```python
from build123d import *

# Parameters (mm, degrees)
SKETCH1_R           = 8.25
BOSS_EXTRUDE1_DEPTH = 85
SKETCH2_OUTSIDE_W   = 36.128
SKETCH2_OUTSIDE_H   = 36.128
SKETCH2_OUTSIDE_R   = 2
CUT_EXTRUDE1_DEPTH  = 12
SKETCH3_R           = 4.75
SKETCH3_R_2         = 4.25
BOSS_EXTRUDE2_DEPTH = 10
CHAMFER1_SIZE       = 1
CHAMFER1_SIZE2      = 3.487414444
FILLET1_R           = 0.5
BOSS_EXTRUDE3_START = -1
SKETCH4_R           = 7.25
BOSS_EXTRUDE3_DEPTH = 1


# Read off the part's stored shape, not the designer's step: Shell1
with BuildPart() as part:
    # Sketch1 → Boss-Extrude1 (new body)
    with BuildSketch(Plane(origin=(0, 0, 0), x_dir=(1, 0, 0), z_dir=(0, 1, 0))):
        with Locations(Location((0, 0, 0), (0, 0, 270))):
            Circle(SKETCH1_R)
    extrude(amount=BOSS_EXTRUDE1_DEPTH)

    # Sketch2 outside → Cut-Extrude1 (cut)
    with BuildSketch(Plane(origin=(0, 85, 0), x_dir=(1, 0, 0), z_dir=(0, 1, 0))):
        Rectangle(SKETCH2_OUTSIDE_W, SKETCH2_OUTSIDE_H)
        with Locations(Location((0, 0, 0), (0, 0, 270))):
            Circle(SKETCH2_OUTSIDE_R, mode=Mode.SUBTRACT)
    extrude(amount=-CUT_EXTRUDE1_DEPTH, mode=Mode.SUBTRACT)

    # Sketch3 → Boss-Extrude2 (add)
    with BuildSketch(Plane(origin=(0, 73, 0), x_dir=(1, 0, 0), z_dir=(0, 1, 0))):
        with Locations(Location((0, 0, 0), (0, 0, 90))):
            Circle(SKETCH3_R)
        with Locations(Location((0, 0, 0), (0, 0, 90))):
            Circle(SKETCH3_R_2, mode=Mode.SUBTRACT)
    extrude(amount=BOSS_EXTRUDE2_DEPTH)

    # Chamfer1
    chamfer1_edges = [part.edges().sort_by_distance(p)[0] for p in [
        (0, 73, -8.25),
    ]]
    chamfer1_side = [part.faces().sort_by_distance(p)[0] for p in [
        (0, 36.5, -8.25),
    ]]
    chamfer(chamfer1_edges, length=CHAMFER1_SIZE, length2=CHAMFER1_SIZE2, reference=chamfer1_side[0])

    # Fillet1
    fillet1_edges = [part.edges().sort_by_distance(p)[0] for p in [
        (0, 72, -8.25),
    ]]
    fillet(fillet1_edges, radius=FILLET1_R)

    # Shell1 outline → Shell1 (revolve, cut)
    with BuildSketch(Plane.XY):
        Polygon((7.25, 0), (7.25, 71.24644595), (4.622044721, 72), (1, 72), (1, 85), (0, 85), (0, 0), align=None)
    revolve(axis=Axis((0, 0, 0), (0, 1, 0)), mode=Mode.SUBTRACT)

    # Sketch4 → Boss-Extrude3 (add)
    with BuildSketch(Plane.XZ.offset(BOSS_EXTRUDE3_START)):
        with BuildLine():
            Line((-13.436556392, 3.352787423), (-6.238581163, 7.278955729))
            ThreePointArc((-6.238581163, 7.278955729), (-3.92093447, 8.189931818), (-1.450059856, 8.5))
            Line((-1.450059856, 8.5), (1.450059856, 8.5))
            ThreePointArc((1.450059856, 8.5), (3.92093447, 8.189931818), (6.238581163, 7.278955729))
            Line((6.238581163, 7.278955729), (13.436556392, 3.352787423))
            ThreePointArc((13.436556392, 3.352787423), (14.579696608, 2.250493995), (15, 0.719100704))
            Line((15, 0.719100704), (15, -0.719100704))
            ThreePointArc((15, -0.719100704), (14.579696608, -2.250493995), (13.436556392, -3.352787423))
            Line((13.436556392, -3.352787423), (6.238581163, -7.278955729))
            ThreePointArc((6.238581163, -7.278955729), (3.92093447, -8.189931818), (1.450059856, -8.5))
            Line((1.450059856, -8.5), (-1.450059856, -8.5))
            ThreePointArc((-1.450059856, -8.5), (-3.92093447, -8.189931818), (-6.238581163, -7.278955729))
            Line((-6.238581163, -7.278955729), (-13.436556392, -3.352787423))
            ThreePointArc((-13.436556392, -3.352787423), (-14.579696608, -2.250493995), (-15, -0.719100704))
            Line((-15, -0.719100704), (-15, 0.719100704))
            ThreePointArc((-15, 0.719100704), (-14.579696608, 2.250493995), (-13.436556392, 3.352787423))
        make_face()
        with Locations(Location((0, 0, 0), (0, 0, 270))):
            Circle(SKETCH4_R, mode=Mode.SUBTRACT)
    extrude(amount=BOSS_EXTRUDE3_DEPTH)


solid = part.part
```
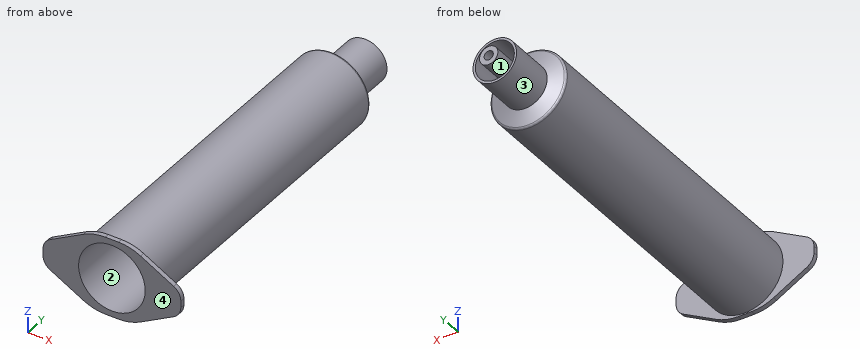
Read the model definition and answer for the solid it produces. Units are mm, in the model's axes. Face numbers are marked on the shaded views. Round coordinates to 2 decimals unless told otherwise and drop trailing zeros. Write each loop counter-clockwise with the first axis right and the second up, starting at its lowest first coordinate (ties: lowest second). Pieces come first, ordered by that corner, then holes. Notation, with made-up numbers: (35, 76) - (73, 76) arc R13 ccw to (73, 80) - close; hole circle Ø4 at (-2, 14). An arc over 180 degrees is marked (long way). Use CSV: the item, a comma, the result in double quotes.
Q1. Find section B-B, the plane x = -12. Write down the section's boundary in (y, z).
Values:
outline,"(0, -4.14) - (1, -4.14) - (1, 4.14) - (0, 4.14) - close"
Q2. Straight lines are drawn through the part: line 1 along X through (y, z) = (77.25, 0); line 2 along X through (y, z) = (53, 0.5); line 3 along Z through (x, y) = (0, 17). For each, find the intervals that lie inside material, in ascending order.
Values:
line 1,"x = -4.75 to -4.25, -2 to -1, 1 to 2, 4.25 to 4.75"
line 2,"x = -8.23 to -7.23, 7.23 to 8.23"
line 3,"z = -8.25 to -7.25, 7.25 to 8.25"
Q3. Determine the mould class of the marked faces 1, 2, 3 and 4 for opening direction X: +X half, -X half, draft (parallel to the pull), parting line (faces both ways), or undercut.
Values:
face 1,"undercut"
face 2,"undercut"
face 3,"parting line"
face 4,"draft"
Q4. Find section A-A, the plane y = 9. Write down the section's boundary in (x, z), then the cut area to 3 significant figures.
Values:
outline,"circle Ø16.5 at (0, 0); hole circle Ø14.5 at (0, 0)"
area,"48.7 mm²"
Q5. Each of these flat-tipped pins is pushed along its axis until it touches: pin 1 Ø8 at (x, z) = (-5, 4) entering from +Y; pin 2 Ø3 at (x, z) = (1.5, -1.5) entering from +Y; pin 3 Ø6 at (y, z) = (47, 6) entering from +X; pin 4 Ø4.5 at (x, z) = (0, 1.5) entering from -Y. Where does it stop, or does it pass through?
Values:
pin 1,"stops at y = 83"
pin 2,"stops at y = 85"
pin 3,"stops at x = 7.69"
pin 4,"stops at y = 72"
